Source: CAD feature listing. Evaluate the final solid. Frame: model axes, mm. Round coordinates to 2 decimals unless told otherwise and drop trailing zeros. Loops run counter-clockwise (first coordinate to the right, second up) from the corner with the lowest first, then second, coordinate; pieces in that order, holes last. Notation, with made-up numbers: M 10,9 L 58,9 A18 ccw 58,30 Z; hole C 26,-17 d6. An arc over 180 degrees is marked long. Answer as a JSON object with one key per item and string values.
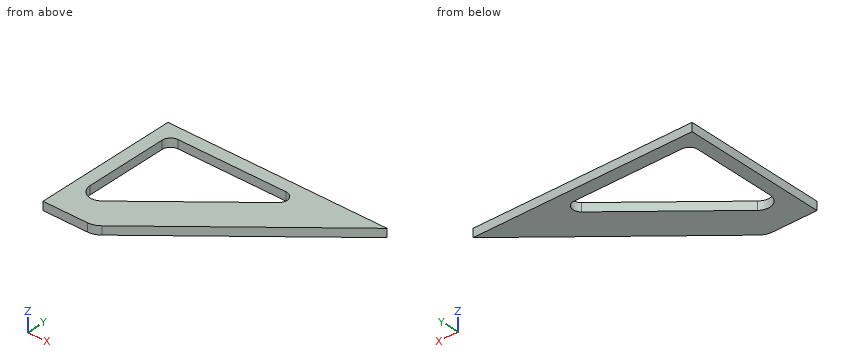
from build123d import *

# Parameters (mm, degrees)
BOSS_EXTRUDE1_DEPTH = 3.175


with BuildPart() as part:
    # Sketch1 → Boss-Extrude1 (new body)
    with BuildSketch(Plane.XY):
        with BuildLine():
            Line((0, 0), (0, -53.7972))
            Line((0, -53.7972), (16.721750646, -53.7972))
            ThreePointArc((16.721750646, -53.7972), (18.907698166, -53.40909009), (20.826436899, -52.292202659))
            Line((20.826436899, -52.292202659), (82.55, 0))
            Line((82.55, 0), (0, 0))
        make_face()
        with BuildLine():
            Line((7.9375, -4.7625), (48.622081998, -4.7625))
            ThreePointArc((48.622081998, -4.7625), (51.603027043, -6.84452624), (50.674425125, -10.36000133))
            Line((50.674425125, -10.36000133), (12.60351469, -42.61367665))
            ThreePointArc((12.60351469, -42.61367665), (7.522504052, -43.300968075), (4.7625, -38.979924656))
            Line((4.7625, -38.979924656), (4.7625, -7.9375))
            ThreePointArc((4.7625, -7.9375), (5.69243597, -5.69243597), (7.9375, -4.7625))
        make_face(mode=Mode.SUBTRACT)
    extrude(amount=BOSS_EXTRUDE1_DEPTH)


solid = part.part
Item 1: Section C-C on y = -30. Return the cut outline in (x, z) (1 decimal).
Answer sheet:
{"outline": "M 0,0 L 4.8,0 L 4.8,3.2 L 0,3.2 Z; M 27.5,0 L 47.1,0 L 47.1,3.2 L 27.5,3.2 Z"}
Item 2: Section A-A on x = 39. Return the cut outline in (y, z) (1 decimal).
Answer sheet:
{"outline": "M -36.9,0 L -20.3,0 L -20.3,3.2 L -36.9,3.2 Z; M -4.8,0 L 0,0 L 0,3.2 L -4.8,3.2 Z"}
Item 3: Section D-D on y = -49.5. Return the cut outline in (x, z) (3 decimals).
Answer sheet:
{"outline": "M 0,0 L 24.122,0 L 24.122,3.175 L 0,3.175 Z"}
Item 4: Contact query for flat-ended pins moving along their axis: pin 1 Ø1 at (y, z) = (-16.5, 1.5) entering from +X; pin 2 Ø1 at (x, z) = (35, 2) entering from -Y; pin 3 Ø1.5 at (y, z) = (-24, 1) entering from +X. Output: stop coordinate, or through.
Answer sheet:
{"pin 1": "stops at x = 63.66", "pin 2": "stops at y = -40.71", "pin 3": "stops at x = 55.11"}
Item 5: Line query: probe 1 along X at (y, z) = (-42.5, 2.3); probe 2 along X at (y, z) = (-33.5, 1.15); probe 3 along Y at (x, z) = (28, 2). Output: solid intervals per line, ascending. Write a range as from..to.
Answer sheet:
{"probe 1": "x = 0..6.32, 12.74..32.38", "probe 2": "x = 0..4.76, 23.36..43.01", "probe 3": "y = -46.21..-29.57, -4.76..0"}
